```python
from build123d import *

# Parameters (mm, degrees)
SKETCH1_R           = 4
BOSS_EXTRUDE1_DEPTH = 100
SKETCH2_R           = 9.096563294
BOSS_EXTRUDE2_DEPTH = 0.254
DOME1_FACE_RADIUS   = 9.096563294
DOME1_HEIGHT        = 5.08
CUT_EXTRUDE1_DEPTH  = 102.076008249
FILLET1_R           = 1.27


with BuildPart() as part:
    # Sketch1 → Boss-Extrude1 (new body)
    with BuildSketch(Plane(origin=(0, 0, 0), x_dir=(1, 0, 0), z_dir=(0, 1, 0))):
        with Locations(Location((0, 0, 0), (0, 0, 270))):
            Circle(SKETCH1_R)
    extrude(amount=BOSS_EXTRUDE1_DEPTH)

    # Sketch2 → Boss-Extrude2 (add)
    with BuildSketch(Plane(origin=(0, 100, 0), x_dir=(1, 0, 0), z_dir=(0, 1, 0))):
        with Locations(Location((0, 0, 0), (0, 0, 270))):
            Circle(SKETCH2_R)
    extrude(amount=BOSS_EXTRUDE2_DEPTH)

    # Dome1: a dome of height H over a round flat face of radius A is a cap of a sphere of radius (A * A + H * H) / (2 * H)
    dome1_r = (DOME1_FACE_RADIUS * DOME1_FACE_RADIUS + DOME1_HEIGHT * DOME1_HEIGHT) / (2 * DOME1_HEIGHT)
    dome1_base = Plane((0, 100.254, 0), z_dir=(0, 1, 0))
    with Locations(dome1_base.offset(DOME1_HEIGHT - dome1_r)):
        dome1_ball = Sphere(dome1_r, mode=Mode.PRIVATE)
    add(split(dome1_ball, bisect_by=dome1_base, keep=Keep.TOP, mode=Mode.PRIVATE))

    # Sketch3 → Cut-Extrude1 (cut, through all)
    with BuildSketch(Plane(origin=(0, 100.254, 0), x_dir=(1, 0, 0), z_dir=(0, 1, 0))):
        Polygon((1.770969394, 5.720489675), (-4.068604684, 4.393949322), (-5.839574078, -1.326540353), (-1.770969394, -5.720489675), (4.068604684, -4.393949322), (5.839574078, 1.326540353), align=None)
    extrude(amount=CUT_EXTRUDE1_DEPTH, mode=Mode.SUBTRACT)

    # Fillet1
    fillet1_edges = [part.edges().sort_by_distance(p)[0] for p in [
        (-4.954089381, 100.254, -1.533704485),
        (-3.805271736, 100.254, 3.523515014),
        (1.148817645, 100.254, 5.057219499),
        (4.954089381, 100.254, 1.533704485),
        (3.805271736, 100.254, -3.523515014),
        (-1.148817645, 100.254, -5.057219499),
    ]]
    fillet(fillet1_edges, radius=FILLET1_R)


solid = part.part
```
Here's how the part is built. I have some questions about the finished solid (model axes, mm). A direction names the side the tool comes from. Give positions to 0.01 mm unless a question says otherwise; leave off trailing zeros. Order: outer loops, then holes, each group sorted by start corner. A loop starts at its lowest first (then second) coordinate and runs counter-clockwise, first axis right, second up. Notation, with made-up numbers: (-21, 0) -> (-6, 0) arc R7 cw to (-6, 4) -> close; hole circle Ø4 at (1.25, 73.25). An arc over 180 degrees is marked (long way). Use CSV: the item, a comma, the result in double quotes. Start each with the question number.
Item 1: On a 3-axis mill with a long thin cutter (end or side, diameter ignored), from which of +Z, -Z, +X, -X, +Y, -Y can I reach the whole of each face in a straight line? I mean faces 1 (the flat face through (3.834, 102.74, -3.493)), 2 (the flat face through (0, 0, 0)), 3 (the flat face through (-2, 100, 4)). Say none if no direction works.
Item 2: I'm going to push flat-ended pins straight in: P1, Ø5, axis at x = -3.5, y = 20.5, coming from the -Z side; P2, Ø8, axis at y = 80, z = 2.5, coming from the -X side; P3, Ø2, axis at x = -7, z = 5.5, coming from the -Y side. Where does each tip first touch, or does it pass through?
Item 3: Suppose I cut it at A-A (y = 95.5). List the corners of the cut face in (x, z) for me, and give its area (3 significant figures).
Item 4: If I drill on probe 1 along Y at (x, z) = (1, -3.25); probe 2 along Y at (x, z) = (-1, -4); probe 3 along X at (y, z) = (15, -2.25), over which ranges is the centre line in solid material (lowest first)? Write a range as [from, to].
Item 5: Suppose I cut it at B-B (x = -7.5). List the corners of the cut face in (y, z) for me.
Answer block:
1,face 1,"+Y"
1,face 2,"+Z, -Z, +X, -X, -Y"
1,face 3,"-Y"
2,P1,"stops at z = -3.87"
2,P2,"stops at x = -4"
2,P3,"stops at y = 100"
3,outline,"circle Ø8 at (0, 0)"
3,area,"50.3 mm^2"
4,probe 1,"y = [0, 100.25]"
4,probe 2,"y = [100, 100.27]"
4,probe 3,"x = [-3.31, 3.31]"
5,outline,"(100, -5.15) -> (100.25, -5.15) arc R7.61 ccw to (100.25, 5.15) -> (100, 5.15) -> close"
